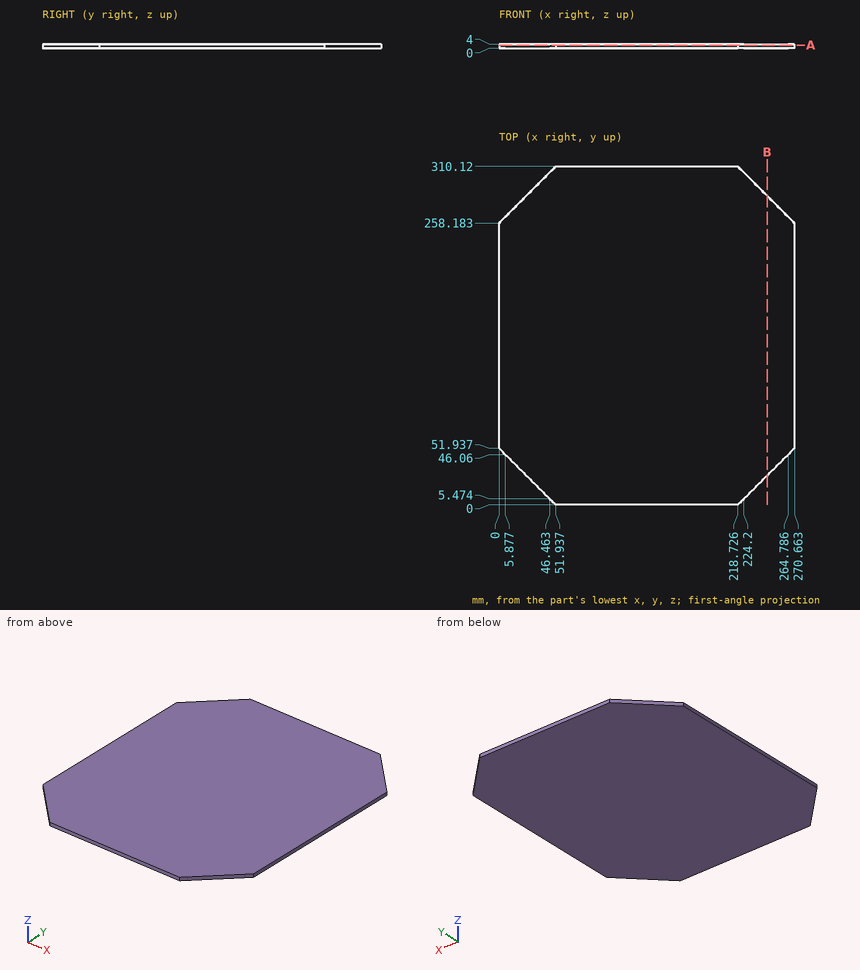
The figure shows three views and two pictorial views of one solid part (mm, origin at its lowest corner). Answer the questions. Give positions to 0.01 mm unless a question says otherwise; leave off trailing zeros. Write each loop counter-clockwise with the first axis right and the second up, starting at its lowest first coordinate (ties: lowest second). Pieces come first, ordered by that corner, then holes. Notation, with made-up numbers: (-24, 62.5) - (-17, 62.5) arc R32 ccw to (-17, 95.5) - close; hole circle Ø9 at (-23.5, 58). An arc over 180 degrees is marked (long way). Use CSV: the item, a comma, the result in double quotes. Start each with the question number.
Item 1: The part is cut by section A-A, the plane z = 3. Give the vertices of the cut face in (x, y), and give its area (3 significant figures).
Item 2: Consider line 1 (X direction, y = 34.5, z = 2.75) (1 decimal); line 2 (X direction, y = 287, z = 1.8) (1 decimal). Determine where each line is inside the solid, lowest interval first.
Item 3: The part is cut by section B-B, the plane x = 245.5. Give the vertices of the cut face in (y, z), and give its area (3 significant figures).
Taken from the geometry:
1,outline,"(0, 51.94) - (51.94, 0) - (218.73, 0) - (270.66, 51.94) - (270.66, 258.18) - (218.73, 310.12) - (51.94, 310.12) - (0, 258.18) - close"
1,area,"78,500 mm2"
2,line 1,"17.4 to 253.2"
2,line 2,"28.8 to 241.8"
3,outline,"(26.77, 0) - (283.35, 0) - (283.35, 4) - (26.77, 4) - close"
3,area,"1,030 mm2"
